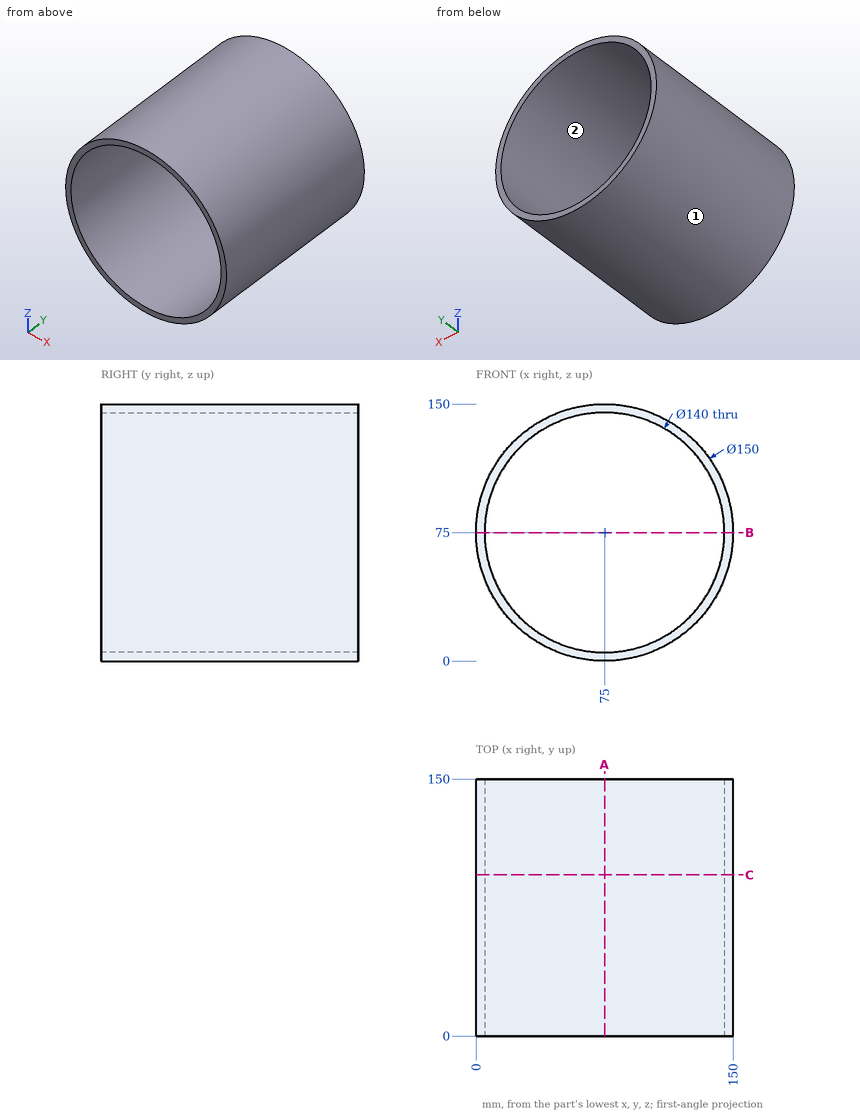
Part print with two shaded views. Sizes in mm from the minimum x, y, z corner. Give positions to 0.01 mm unless a question says otherwise; leave off trailing zeros. Order: outer loops, then holes, each group sorted by start corner. A loop starts at its lowest first (then second) coordinate and runs counter-clockwise, first axis right, second up. Notation, with made-up numbers: M -2.5,-12 L 10.5,-12 A6 ccw 10.5,-1 Z; hole C 75.5,56.25 d2. An arc over 180 degrees is marked long. Write item = value, one per line.
Q1. Flat gauge pins, fed straight in: pin 1 (1 mm diameter, centred on y = 76, z = 99.5, fed in from +X); pin 2 (12 mm diameter, centred on x = 62.5, y = 92, fed in from +Z); pin 3 (1 mm diameter, centred on y = 127.5, z = 62.5, fed in from -X). Where does each tip first touch, or does it go through?
Derived:
pin_1 = 146.06
pin_2 = 149.72
pin_3 = 0.97
Q2. Cut at C-C, the plane y = 94. List the corners of the cut face in (x, z), then the cut area to 3 significant figures.
Derived:
outline = C 75,75 d150; hole C 75,75 d140
area = 2,280 mm2
Q3. Cut at A-A, the plane x = 75. List the corners of the cut face in (y, z), then the cut area to 3 significant figures.
Derived:
outline = M 0,0 L 150,0 L 150,5 L 0,5 Z; M 0,145 L 150,145 L 150,150 L 0,150 Z
area = 1,500 mm2
Q4. Drill centre lines: line 1 (Z direction, x = 77.5, y = 28.5); line 2 (X direction, y = 100.5, z = 75); line 3 (X direction, y = 21, z = 99). Where is each one in solid material? Low to high. Write a range as [from, to].
Derived:
line_1 = [0.04, 5.04], [144.96, 149.96]
line_2 = [0, 5], [145, 150]
line_3 = [3.94, 9.24], [140.76, 146.06]
Q5. Cut at B-B, the plane z = 75. List the corners of the cut face in (x, y).
Derived:
outline = M 0,0 L 5,0 L 5,150 L 0,150 Z; M 145,0 L 150,0 L 150,150 L 145,150 Z
Q6. Two-plate mould, pull along X, no slides. Class the marked faces 1 and 2: pulls with the +X half, pulls with the -X half, needs draft (parallel to the pull), parting line crosses it, or undercut.
Derived:
face_1 = parting line crosses it
face_2 = undercut
